```python
from build123d import *

# Parameters (mm, degrees)
SKETCH1_W                = 26.67
SKETCH1_H                = 10.668
BOSS_EXTRUDE1_DEPTH      = 0.254
EXTRUDE_THIN1_DEPTH      = 0.254
EXTRUDE_THIN1_DEPTH_BACK = 2.921
SKETCH1_3_W              = 27.686
SKETCH1_3_H              = 11.684
SKETCH1_3_W_2            = 26.67
SKETCH1_3_H_2            = 10.668
SKETCH5_W                = 1.27
SKETCH5_H                = 11.684
BOSS_EXTRUDE2_DEPTH      = 3.683
CUT_EXTRUDE1_DEPTH       = 31.975766028
LPATTERN1_COUNT          = 4
LPATTERN1_PITCH          = 2.54
CUT_EXTRUDE2_DEPTH       = 20.408159779


with BuildPart() as part:
    # Sketch1 → Boss-Extrude1 (new body)
    with BuildSketch(Plane(origin=(0, 0, 0), x_dir=(0, 0, -1), z_dir=(1, 0, 0))):
        Rectangle(SKETCH1_W, SKETCH1_H)
    extrude(amount=BOSS_EXTRUDE1_DEPTH)

    # Sketch1<3> → Extrude-Thin1 (add, two sides: drawn at the far end of the back side and taken through both)
    with BuildSketch(Plane(origin=(0, 0, 0), x_dir=(0, 0, -1), z_dir=(1, 0, 0)).offset(-EXTRUDE_THIN1_DEPTH_BACK)):
        Rectangle(SKETCH1_3_W, SKETCH1_3_H)
        Rectangle(SKETCH1_3_W_2, SKETCH1_3_H_2, mode=Mode.SUBTRACT)
    extrude(amount=EXTRUDE_THIN1_DEPTH + EXTRUDE_THIN1_DEPTH_BACK)

    # Sweep1: sweep along a path in Sketch2
    with BuildLine(Plane.ZY.offset(2.921)) as sweep1_path:
        Line((-13.335, -5.334), (13.335, -5.334))
        Line((13.335, -5.334), (13.335, 5.334))
        Line((13.335, 5.334), (-13.335, 5.334))
        Line((-13.335, 5.334), (-13.335, -5.334))
    # Sketch3 → Sweep1 (sweep)
    with BuildSketch(Plane(origin=(0, 0, 0), x_dir=(-1, 0, 0), z_dir=(0, -1, 0))):
        Polygon((2.921, -13.335), (3.140970453, -12.954), (3.429, -13.242029547), (3.429, -13.843), (2.921, -13.843), align=None)
    sweep(path=sweep1_path.line, transition=Transition.RIGHT)

    # Sketch5 → Boss-Extrude2 (add)
    with BuildSketch(Plane.ZY.offset(3.429)):
        with Locations((-14.478, 0)):
            Rectangle(SKETCH5_W, SKETCH5_H)
        with Locations((14.478, 0)):
            Rectangle(SKETCH5_W, SKETCH5_H)
    extrude(amount=-BOSS_EXTRUDE2_DEPTH)

    # Sketch4 → Cut-Extrude1 (cut, symmetric)
    with BuildSketch(Plane.XY.offset(15.113)):
        with BuildLine():
            Line((-1.27, 4.572), (-3.429, 4.572))
            Line((-3.429, 4.572), (-3.429, 3.048))
            Line((-3.429, 3.048), (-1.27, 3.048))
            ThreePointArc((-1.27, 3.048), (-0.508, 3.81), (-1.27, 4.572))
        make_face()
    cut_extrude1 = extrude(amount=CUT_EXTRUDE1_DEPTH, both=True, mode=Mode.SUBTRACT)

    # LPattern1: Cut-Extrude1 ×4
    with Locations(*[(0, -i * LPATTERN1_PITCH, 0) for i in range(1, LPATTERN1_COUNT)]):
        add(cut_extrude1, mode=Mode.SUBTRACT)

    # Sketch7 → Cut-Extrude2 (cut, through all)
    with BuildSketch(Plane.XZ.offset(5.842)):
        Polygon((-3.429, 8.255), (-1.905, 6.731), (-1.905, -6.731), (-3.429, -8.255), align=None)
    extrude(amount=-CUT_EXTRUDE2_DEPTH, mode=Mode.SUBTRACT)


solid = part.part
```
For this review, take the finished solid that the model builds, in its own axes (mm). A direction names the side the tool comes from. Round coordinates to 2 decimals unless told otherwise and drop trailing zeros. Write each loop counter-clockwise with the first axis right and the second up, starting at its lowest first coordinate (ties: lowest second). Pieces come first, ordered by that corner, then holes. Notation, with made-up numbers: (7.5, 69.5) -> (63.5, 69.5) arc R20 cw to (63.5, 102.5) -> close; hole circle Ø6 at (3.5, 62.25). An arc over 180 degrees is marked (long way). One line per question, with ' | ' between items. Start each with the question number.
(1) Add section C-C, the plane x = -2.55. Give the number of separate pieces and of enclosed holes in the cut face, plus the area to 3 significant figures.
(2) Tool access review of faces 1 (the face through (-2.656, -5.503, -7.482)), 2 (the face through (-2, 4.572, 14)), 3 (the face through (-3.429, 5.4, -12.5)): name each direction out of +Z, -Z, +X, -X, +Y, -Y from which nothing blocks a thin tool from reaching the whole face with its end or side.
(3) Add section A-A, the plane z = -5. Write out the cut boundary in (x, y) (3 decimals).
(4) Insertion check: P1, Ø4, axis at y = -1.5, z = -9, coming from the -X side. The pin has a flat end and moves straight along its axis. Give the tip position at first contact, or say it passes through.
(5) For line 1 along Z through (x, y) = (-2.4, 2.5) (3 decimals); line 2 along Y through (x, z) = (-2.4, 8.5); line 3 along X through (y, z) = (-3, -4.5), list the stretches that pass through material, from the lowest coordinate up. Write a range as from..to.
(6) Add section B-B, the plane y = -3.81. Write out the cut boundary in (x, z) (3 decimals), plus the area to 3 significant figures.
(7) Add section D-D, the plane z = -11. Write out the cut boundary in (x, y).
(8) Mouldability with a two-part tool opening along X and no side actions: class faces 4 (the face through (-1, 0, 13.335)), 5 (the face through (-2, 2.032, -14)), 6 (the face through (-3.429, 2.5, -14.2)), 7 (the face through (-1, -5.334, 0)) as released by +X, released by -X, zero draft, split by the parting line, or undercut.
Answer list:
1) separate pieces: 10 | enclosed holes: 0 | area: 32.0 mm²
2) face 1: -X, +Y, -Y | face 2: +Z, -Z, -X | face 3: +Z, -Z, -X, +Y, -Y
3) outline: (-1.905, -5.842) -> (0.254, -5.842) -> (0.254, 5.842) -> (-1.905, 5.842) -> (-1.905, 5.334) -> (0, 5.334) -> (0, -5.334) -> (-1.905, -5.334) -> close
4) P1: x = 0
5) line 1: -15.113..-13.335, 13.335..15.113 | line 2: -5.84..-5.33, 5.33..5.84 | line 3: 0..0.25
6) outline: (-0.508, -15.113) -> (0.254, -15.113) -> (0.254, 15.113) -> (-0.508, 15.113) -> (-0.508, 13.335) -> (0, 13.335) -> (0, -13.335) -> (-0.508, -13.335) -> close | area: 9.48 mm²
7) outline: (-3.43, -5.84) -> (0.25, -5.84) -> (0.25, 5.84) -> (-3.43, 5.84) -> (-3.43, 5.24) -> (-3.14, 4.95) -> (-2.92, 5.33) -> (0, 5.33) -> (0, -5.33) -> (-2.92, -5.33) -> (-3.14, -4.95) -> (-3.43, -5.24) -> close
8) face 4: undercut | face 5: zero draft | face 6: released by -X | face 7: undercut
